The listing builds one solid part. Answer for the finished solid, in the listing's coordinates (mm). Face numbers are marked on the shaded views. A direction names the side the tool comes from. Round coordinates to 2 decimals unless told otherwise and drop trailing zeros. Loops run counter-clockwise (first coordinate to the right, second up) from the corner with the lowest first, then second, coordinate; pieces in that order, holes last. Notation, with made-up numbers: M -32,-23 L 12,-23 A24 ccw 12,7 Z; hole C 60.25,49 d3. An arc over 180 degrees is marked long. Answer as a JSON object with one key per item and string values.
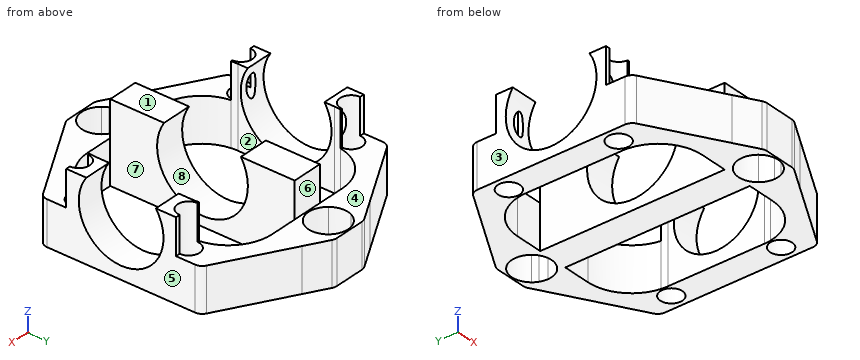
```python
from build123d import *

# Parameters (mm, degrees)
BOSS_EXTRUDE1_DEPTH = 12.7
SKETCH1_4_W         = 8.808271716
SKETCH1_4_H         = 53.34
BOSS_EXTRUDE3_DEPTH = 23
CUT_EXTRUDE3_REACH  = 82.003
SKETCH9_R           = 13.125
CUT_EXTRUDE4_REACH  = 82.003
SKETCH8_R           = 12.25


with BuildPart() as part:
    # Sketch1 → Boss-Extrude1 (new body)
    with BuildSketch(Plane.XY):
        with BuildLine():
            Line((4.404135858, -36.408089009), (4.404135858, -38.862))
            ThreePointArc((4.404135858, -38.862), (5.057273366, -38.776589863), (5.666486021, -38.52610346))
            Line((5.666486021, -38.52610346), (11.954126984, -34.925))
            Line((11.954126984, -34.925), (5.291497331, -34.925))
            ThreePointArc((5.291497331, -34.925), (4.904203705, -35.700282028), (4.404135858, -36.408089009))
        make_face()
        with BuildLine():
            Line((-4.404135858, -36.408089009), (-4.404135858, -38.862))
            Line((-4.404135858, -38.862), (4.404135858, -38.862))
            Line((4.404135858, -38.862), (4.404135858, -36.408089009))
            ThreePointArc((4.404135858, -36.408089009), (0, -38.481), (-4.404135858, -36.408089009))
        make_face()
        with BuildLine():
            Line((4.404135858, -26.67), (4.404135858, -29.123910991))
            ThreePointArc((4.404135858, -29.123910991), (5.377307013, -30.830594542), (5.715, -32.766))
            ThreePointArc((5.715, -32.766), (5.60812501, -33.866072215), (5.291497331, -34.925))
            Line((5.291497331, -34.925), (11.954126984, -34.925))
            Line((11.954126984, -34.925), (31.742350164, -23.591744906))
            ThreePointArc((31.742350164, -23.591744906), (32.677495098, -22.661460621), (33.02, -21.387641446))
            Line((33.02, -21.387641446), (33.02, -15.875))
            Line((33.02, -15.875), (31.75, -15.875))
            ThreePointArc((31.75, -15.875), (28.575, -19.05), (25.4, -15.875))
            Line((25.4, -15.875), (24.875312158, -15.875))
            ThreePointArc((24.875312158, -15.875), (20.598387055, -23.600251814), (12.319, -26.67))
            Line((12.319, -26.67), (4.404135858, -26.67))
        make_face()
        with BuildLine():
            Line((-33.02, -15.875), (-33.02, -21.387641446))
            ThreePointArc((-33.02, -21.387641446), (-32.677495098, -22.661460621), (-31.742350164, -23.591744906))
            Line((-31.742350164, -23.591744906), (-11.954126984, -34.925))
            Line((-11.954126984, -34.925), (-5.291497331, -34.925))
            ThreePointArc((-5.291497331, -34.925), (-5.649290588, -31.901858317), (-4.404135858, -29.123910991))
            Line((-4.404135858, -29.123910991), (-4.404135858, -26.67))
            Line((-4.404135858, -26.67), (-12.319, -26.67))
            ThreePointArc((-12.319, -26.67), (-20.598387055, -23.600251814), (-24.875312158, -15.875))
            Line((-24.875312158, -15.875), (-25.4, -15.875))
            ThreePointArc((-25.4, -15.875), (-28.575, -19.05), (-31.75, -15.875))
            Line((-31.75, -15.875), (-33.02, -15.875))
        make_face()
        with BuildLine():
            Line((-5.291497331, -34.925), (-11.954126984, -34.925))
            Line((-11.954126984, -34.925), (-5.666486021, -38.52610346))
            ThreePointArc((-5.666486021, -38.52610346), (-5.057273366, -38.776589863), (-4.404135858, -38.862))
            Line((-4.404135858, -38.862), (-4.404135858, -36.408089009))
            ThreePointArc((-4.404135858, -36.408089009), (-4.904203705, -35.700282028), (-5.291497331, -34.925))
        make_face()
        with BuildLine():
            Line((-4.404135858, -26.67), (-4.404135858, -29.123910991))
            ThreePointArc((-4.404135858, -29.123910991), (0, -27.051), (4.404135858, -29.123910991))
            Line((4.404135858, -29.123910991), (4.404135858, -26.67))
            Line((4.404135858, -26.67), (-4.404135858, -26.67))
        make_face()
        with BuildLine():
            Line((4.404135858, 29.123910991), (4.404135858, 26.67))
            Line((4.404135858, 26.67), (12.319, 26.67))
            ThreePointArc((12.319, 26.67), (20.598387055, 23.600251814), (24.875312158, 15.875))
            Line((24.875312158, 15.875), (25.4, 15.875))
            ThreePointArc((25.4, 15.875), (28.575, 19.05), (31.75, 15.875))
            Line((31.75, 15.875), (33.02, 15.875))
            Line((33.02, 15.875), (33.02, 21.387641446))
            ThreePointArc((33.02, 21.387641446), (32.677495098, 22.661460621), (31.742350164, 23.591744906))
            Line((31.742350164, 23.591744906), (11.954126984, 34.925))
            Line((11.954126984, 34.925), (5.291497331, 34.925))
            ThreePointArc((5.291497331, 34.925), (5.60812501, 33.866072215), (5.715, 32.766))
            ThreePointArc((5.715, 32.766), (5.377307013, 30.830594542), (4.404135858, 29.123910991))
        make_face()
        with BuildLine():
            ThreePointArc((5.666486021, 38.52610346), (5.057273366, 38.776589863), (4.404135858, 38.862))
            Line((4.404135858, 38.862), (4.404135858, 36.408089009))
            ThreePointArc((4.404135858, 36.408089009), (4.904203705, 35.700282028), (5.291497331, 34.925))
            Line((5.291497331, 34.925), (11.954126984, 34.925))
            Line((11.954126984, 34.925), (5.666486021, 38.52610346))
        make_face()
        with BuildLine():
            Line((4.404135858, 38.862), (-4.404135858, 38.862))
            Line((-4.404135858, 38.862), (-4.404135858, 36.408089009))
            ThreePointArc((-4.404135858, 36.408089009), (0, 38.481), (4.404135858, 36.408089009))
            Line((4.404135858, 36.408089009), (4.404135858, 38.862))
        make_face()
        with BuildLine():
            Line((-33.02, 21.387641446), (-33.02, 15.875))
            Line((-33.02, 15.875), (-31.75, 15.875))
            ThreePointArc((-31.75, 15.875), (-28.575, 19.05), (-25.4, 15.875))
            Line((-25.4, 15.875), (-24.875312158, 15.875))
            ThreePointArc((-24.875312158, 15.875), (-20.598387055, 23.600251814), (-12.319, 26.67))
            Line((-12.319, 26.67), (-4.404135858, 26.67))
            Line((-4.404135858, 26.67), (-4.404135858, 29.123910991))
            ThreePointArc((-4.404135858, 29.123910991), (-5.649290588, 31.901858317), (-5.291497331, 34.925))
            Line((-5.291497331, 34.925), (-11.954126984, 34.925))
            Line((-11.954126984, 34.925), (-31.742350164, 23.591744906))
            ThreePointArc((-31.742350164, 23.591744906), (-32.677495098, 22.661460621), (-33.02, 21.387641446))
        make_face()
        with BuildLine():
            Line((-5.666486021, 38.52610346), (-11.954126984, 34.925))
            Line((-11.954126984, 34.925), (-5.291497331, 34.925))
            ThreePointArc((-5.291497331, 34.925), (-4.904203705, 35.700282028), (-4.404135858, 36.408089009))
            Line((-4.404135858, 36.408089009), (-4.404135858, 38.862))
            ThreePointArc((-4.404135858, 38.862), (-5.057273366, 38.776589863), (-5.666486021, 38.52610346))
        make_face()
        with BuildLine():
            Line((-4.404135858, 29.123910991), (-4.404135858, 26.67))
            Line((-4.404135858, 26.67), (4.404135858, 26.67))
            Line((4.404135858, 26.67), (4.404135858, 29.123910991))
            ThreePointArc((4.404135858, 29.123910991), (0, 27.051), (-4.404135858, 29.123910991))
        make_face()
    extrude(amount=BOSS_EXTRUDE1_DEPTH)

    # Sketch1<4> → Boss-Extrude3 (add)
    with BuildSketch(Plane.XY):
        with BuildLine():
            ThreePointArc((25.019, -13.97), (24.983027093, -14.925205632), (24.875312158, -15.875))
            Line((24.875312158, -15.875), (25.4, -15.875))
            ThreePointArc((25.4, -15.875), (28.575, -12.7), (31.75, -15.875))
            Line((31.75, -15.875), (33.02, -15.875))
            Line((33.02, -15.875), (33.02, 15.875))
            Line((33.02, 15.875), (31.75, 15.875))
            ThreePointArc((31.75, 15.875), (28.575, 12.7), (25.4, 15.875))
            Line((25.4, 15.875), (24.875312158, 15.875))
            ThreePointArc((24.875312158, 15.875), (24.983027093, 14.925205632), (25.019, 13.97))
            Line((25.019, 13.97), (25.019, -13.97))
        make_face()
        with BuildLine():
            Line((-33.02, 15.875), (-33.02, -15.875))
            Line((-33.02, -15.875), (-31.75, -15.875))
            ThreePointArc((-31.75, -15.875), (-28.575, -12.7), (-25.4, -15.875))
            Line((-25.4, -15.875), (-24.875312158, -15.875))
            ThreePointArc((-24.875312158, -15.875), (-24.983027093, -14.925205632), (-25.019, -13.97))
            Line((-25.019, -13.97), (-25.019, 13.97))
            ThreePointArc((-25.019, 13.97), (-24.983027093, 14.925205632), (-24.875312158, 15.875))
            Line((-24.875312158, 15.875), (-25.4, 15.875))
            ThreePointArc((-25.4, 15.875), (-28.575, 12.7), (-31.75, 15.875))
            Line((-31.75, 15.875), (-33.02, 15.875))
        make_face()
        Rectangle(SKETCH1_4_W, SKETCH1_4_H)
    extrude(amount=BOSS_EXTRUDE3_DEPTH)

    # Cut-Extrude3: up to this face of the body (flat: up to its plane)
    cut_extrude3_end = Plane(part.part.faces().sort_by_distance((4.404135858, 0, 11.5))[0])
    # Sketch9 → Cut-Extrude3 (cut, up to the picked face)
    with BuildSketch(Plane.ZY.offset(33.02), mode=Mode.PRIVATE) as cut_extrude3_sk1:
        with Locations((16, 0)):
            Circle(SKETCH9_R)
    cut_extrude3_tool1 = split(extrude(cut_extrude3_sk1.sketch, amount=-CUT_EXTRUDE3_REACH, mode=Mode.PRIVATE), bisect_by=cut_extrude3_end, keep=Keep.BOTH, mode=Mode.PRIVATE)
    add(cut_extrude3_tool1.solids().sort_by(Axis((-33.02, 0, 16), (1, 0, 0)))[0], mode=Mode.SUBTRACT)

    # Sketch8 → Cut-Extrude4 (cut, up to next)
    with BuildSketch(Plane(origin=(33.02, 0, 0), x_dir=(0, 0, -1), z_dir=(1, 0, 0)), mode=Mode.PRIVATE) as cut_extrude4_sk1:
        with Locations((-16, 0)):
            Circle(SKETCH8_R)
    cut_extrude4_tool1 = extrude(cut_extrude4_sk1.sketch, amount=-CUT_EXTRUDE4_REACH, mode=Mode.PRIVATE) & part.part
    add(cut_extrude4_tool1.solids().sort_by_distance((33.02, 0, 16))[0], mode=Mode.SUBTRACT)


solid = part.part
```
Item 1: The part is cut by section C-C (x = -23). Give the vertices of the cut face in (y, z).
Values follow:
{"outline": "M -28.6,0 L -20.84,0 L -20.84,12.7 L -28.6,12.7 Z; M 20.84,0 L 28.6,0 L 28.6,12.7 L 20.84,12.7 Z"}
Item 2: Determine the mould class of the marked faces 1, 2 and 3 for opening direction X: released by +X, released by -X, zero draft, split by the parting line, or undercut.
Values follow:
{"face 1": "zero draft", "face 2": "undercut", "face 3": "released by -X"}
Item 3: Straight lines are drawn through the part: line 1 (X direction, y = 6.5, z = 3); line 2 (Y direction, x = -1.5, z = 16) (3 decimals); line 3 (Y direction, x = 30, z = 3.5). For each, find the intervals that lie inside material, in ascending order.
Values follow:
{"line 1": "-33.02 to -25.02, -4.4 to 4.4, 25.02 to 33.02", "line 2": "-26.67 to -13.125, 13.125 to 26.67", "line 3": "-24.59 to -18.71, -13.04 to 13.04, 18.71 to 24.59"}
Item 4: The part is cut by section B-B (y = 0). Give the vertices of the cut face in (x, z) (3 decimals), then the cut area to 3 significant figures.
Values follow:
{"outline": "M -33.02,0 L -25.019,0 L -25.019,2.875 L -33.02,2.875 Z; M -4.404,0 L 4.404,0 L 4.404,2.875 L -4.404,2.875 Z; M 25.019,0 L 33.02,0 L 33.02,3.75 L 25.019,3.75 Z", "area": "78.3 mm^2"}
Item 5: The part is cut by section D-D (y = 30). Give the vertices of the cut face in (x, z).
Values follow:
{"outline": "M -20.55,0 L -5,0 L -5,12.7 L -20.55,12.7 Z; M 5,0 L 20.55,0 L 20.55,12.7 L 5,12.7 Z"}
Item 6: The part is cut by section A-A (x = 0). Give the number of separate pieces and of enclosed holes in the cut face, then the cut area to 3 significant figures.
Values follow:
{"separate pieces": "3", "enclosed holes": "0", "area": "801 mm^2"}
Item 7: Which of the six approach directions +Z, -Z, +X, -X, +Y, -Y give full straight-line access (tool end or side, diameter ignored) to the marked faces 4, 5, 6, 7 and 8?
Values follow:
{"face 4": "+Z, +Y", "face 5": "+Z, -Z, +X, +Y, -Y", "face 6": "+Z, +X, -X, +Y", "face 7": "+Z, -Z", "face 8": "-X"}
Item 8: Flat-ended cylindrical pins translate along their axes: P1, Ø1, axis at x = 32.5, z = 19.5, coming from the -Y side (3 decimals); P2, Ø4.5, axis at x = -2, z = 19, coming from the +Y side; P3, Ø1, axis at x = -32, z = 16, coming from the +Y side (3 decimals). Find the tip coordinate at first contact, or state that the pin passes through.
Values follow:
{"P1": "y = -15.875", "P2": "y = 26.67", "P3": "y = 15.875"}
